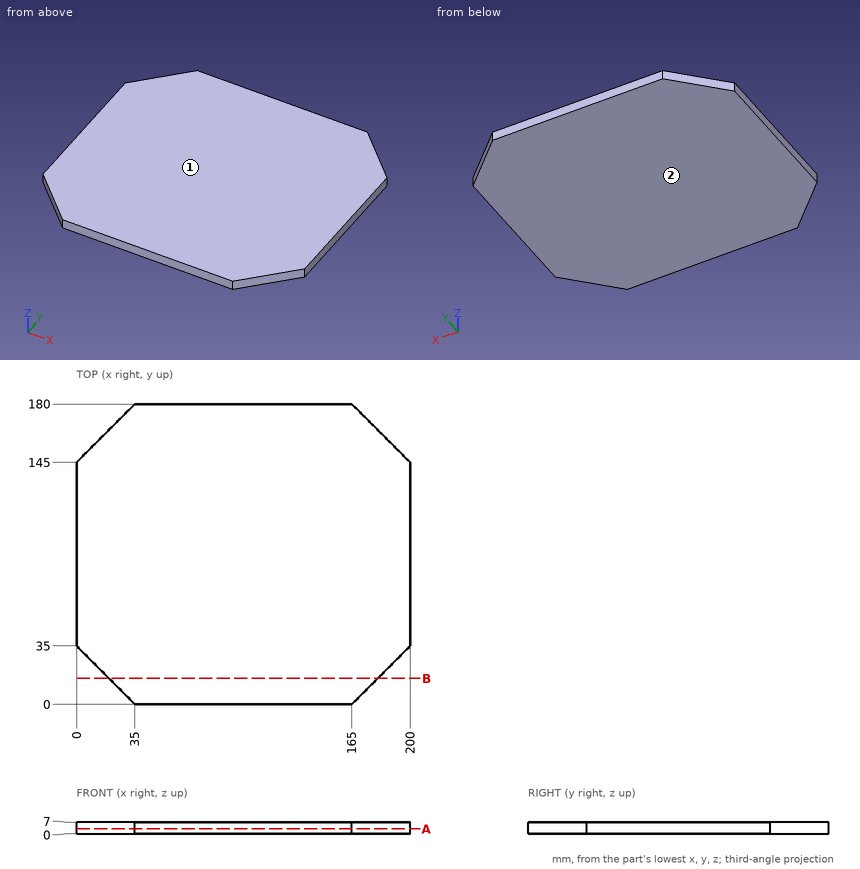
Drawing for the job (mm, zero at the part's lowest x, y, z). Round coordinates to 2 decimals unless told otherwise and drop trailing zeros. Write each loop counter-clockwise with the first axis right and the second up, starting at its lowest first coordinate (ties: lowest second). Pieces come first, ordered by that corner, then holes. Notation, with made-up numbers: (-12, 69.5) - (-5, 69.5) arc R27 cw to (-5, 105.5) - close; hole circle Ø9 at (31.25, -4.5). An arc over 180 degrees is marked (long way). Return JSON: item names as keys, results as strings. Group by question number.
Item 1: Mould opens along Z. For the marked faces 1 and 2 say: +Z half, -Z half, draft (parallel to the pull), parting line (faces both ways), or undercut.
Item 2: Band-saw the part on B-B on y = 15.5. List the corners of the cut face in (x, z).
Item 3: Probe probe 1 along X at (y, z) = (173, 2); probe 2 along X at (y, z) = (31.5, 6.75); probe 3 along Y at (x, z) = (30.5, 2.5). List the from-to ranges inside material, lowest first.
Item 4: Band-saw the part on A-A on z = 3. List the corners of the cut face in (x, y).
Item 5: Flat gauge pins, fed straight in: pin 1 Ø1.5 at (x, z) = (20.5, 1) entering from -Y; pin 2 Ø4 at (y, z) = (32.5, 4.5) entering from -X. Where does each tip first touch, or does it go through?
Resolved:
{
 "1": {"face 1": "+Z half", "face 2": "-Z half"},
 "2": {"outline": "(19.5, 0) - (180.5, 0) - (180.5, 7) - (19.5, 7) - close"},
 "3": {"probe 1": "x = 28 to 172", "probe 2": "x = 3.5 to 196.5", "probe 3": "y = 4.5 to 175.5"},
 "4": {"outline": "(0, 35) - (35, 0) - (165, 0) - (200, 35) - (200, 145) - (165, 180) - (35, 180) - (0, 145) - close"},
 "5": {"pin 1": "stops at y = 13.75", "pin 2": "stops at x = 0.5"}
}
